Part model, mm, in its own coordinate system. Face numbers are marked on the shaded views. A direction names the side the tool comes from. Coordinates: 2 decimals unless noted, no trailing zeros. Write each loop counter-clockwise with the first axis right and the second up, starting at its lowest first coordinate (ties: lowest second). Pieces come first, ordered by that corner, then holes. Notation, with made-up numbers: (5.5, 9.25) -> (9.5, 9.25) arc R21 ccw to (9.5, 32.25) -> close; hole circle Ø7 at (55, -38.75). An arc over 180 degrees is marked (long way). Write item = value, one per line.
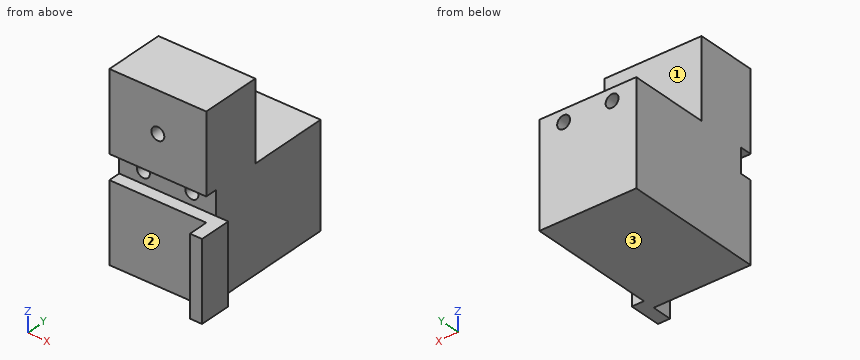
Autodesk Inventor part; units mm, degrees
ref_plane "YZ Plane" through (0, 0, 0) normal (1, 0, 0) x (0, 1, 0)
ref_plane "XZ Plane" through (0, 0, 0) normal (0, 1, 0) x (-1, 0, 0)
ref_plane "XY Plane" through (0, 0, 0) normal (0, 0, 1) x (1, 0, 0)
sketch "Sketch2" plane through (0, 0, 0) normal (0, 1, 0) x (-1, 0, 0)
  line L0 (12, 22.5) -> (-12, 22.5)
  line L1 (-12, 22.5) -> (-12, -22.5)
  line L2 (-12, -22.5) -> (12, -22.5)
  line L3 (12, -22.5) -> (12, 22.5)
  line L4 (12, 22.5) -> (12, 12.5)
  line L5 (12, 12.5) -> (0, 12.5)
  circle A0 centre (0, 12.5) radius 1.6
  line L6 (0, 12.5) -> (0, 0)
  line L7 (0, 0) -> (-6, 0)
  line L8 (-6, 0) -> (6, 0)
  circle A1 centre (-6, 0) radius 1.6
  circle A2 centre (6, 0) radius 1.6
  line L9 (-12, 22.5) -> (12, 22.5)
  line L10 (12, 22.5) -> (12, 0)
  line L11 (12, 0) -> (-12, 0)
  line L12 (-12, 0) -> (-12, 22.5)
  line L13 (-12, 22.5) -> (12, 22.5)
  line L14 (12, 22.5) -> (12, 2.2056)
  line L15 (12, 2.2056) -> (-12, 2.2056)
  line L16 (-12, 2.2056) -> (-12, 22.5)
  dimension "d0" = 24
  dimension "d1" = 45
  dimension "d2" = 10
  dimension "d3" = 3.2
  dimension "d6" = 6
  dimension "d7" = 3.2
  dimension "d8" = 3.2
extrude "Extrusion1" add sketch "Sketch2" along normal blind 35 contours L3 L5 A0 L6 L15 L1 L0 | L3 L15 L6 A0 L5 | L15 L6 L7 A1 L11 L1 | L3 L11 A2 L8 L6 L15 | L11 A1 L7 L8 A2 L3 L2 L1 | L11 L7 A1 | A1 L7 L11 | L11 L8 A2 | A2 L8 L11
sketch "Sketch3" plane through (0, 0, 0) normal (0, -1, 0) x (1, 0, 0)
  line L0 (12, 22.5) -> (12, -22.5)
  line L1 (-12, -22.5) -> (-12, 22.5)
  line L2 (12, 3) -> (-12, 3)
  line L3 (-12, 3) -> (-12, -3)
  line L4 (-12, -3) -> (12, -3)
  line L5 (12, -3) -> (12, 3)
  point P0 (0, 0)
  dimension "d9" = 6
extrude "Extrusion2" cut sketch "Sketch3" against normal blind 3
hole "Hole1" at (-6, 0, 0) at (6, 0, 0) direction (0, 1, 0) diameter 3.2 depth 44.75 countersink diameter 4 countersink angle 90
sketch "Sketch4" plane through (0, 35, 0) normal (0, 1, 0) x (1, 0, 0)
  line L0 (12, -3) -> (12, 3)
  line L1 (-12, -22.5) -> (12, -22.5)
  line L2 (12, -22.5) -> (12, -3)
  line L3 (12, -3) -> (-12, -3)
  line L4 (-12, -3) -> (-12, -22.5)
  point P0 (0, 0)
extrude "Extrusion3" cut sketch "Sketch4" against normal blind 20
sketch "Sketch5" plane through (12, 0, -22.5) normal (1, 0, 0) x (0, 0, -1)
  line L0 (-45, 0) -> (-25.5, 0)
  line L1 (-45, 0) -> (-45, 15)
  line L2 (-25.5, 0) -> (-45, 0)
  line L3 (-45, 0) -> (-45, 3)
  line L4 (-45, 3) -> (-25.5, 3)
  line L5 (-25.5, 3) -> (-25.5, 0)
  point P0 (-22.5, 0)
  dimension "d21" = 3
extrude "Extrusion4" add sketch "Sketch5" along normal blind 3
sketch "Sketch6" plane through (0, 0, 0) normal (0, -1, 0) x (1, 0, 0)
  line L0 (-12, 3) -> (15, 3)
  line L1 (12, 22.5) -> (12, 3)
  line L2 (15, 3) -> (12, 3)
  line L3 (12, 3) -> (12, 22.5)
  line L4 (12, 22.5) -> (15, 22.5)
  line L5 (15, 22.5) -> (15, 3)
  point P0 (0, 0)
extrude "Extrusion5" add sketch "Sketch6" along normal blind 5
sketch "Sketch7" plane through (-12, 0, 3) normal (0, 0, -1) x (-1, 0, 0)
  line L0 (-24, 0) -> (-24, -5)
  line L1 (-27, 3) -> (-27, -5)
  line L2 (-24, -5) -> (-27, -5)
  line L3 (-27, -5) -> (-27, 3)
  line L4 (-27, 3) -> (-24, 3)
  line L5 (-24, 3) -> (-24, -5)
  point P0 (-12, 0)
extrude "Extrusion6" add sketch "Sketch7" along normal blind 25.5
sketch "Sketch8" plane through (-12, 15, 22.5) normal (0, 0, 1) x (1, 0, 0)
  line L0 (27, -12) -> (27, -20)
  line L1 (24, -12) -> (24, -15)
  line L2 (27, -20) -> (24, -20)
  line L3 (24, -20) -> (24, -12)
  line L4 (24, -12) -> (27, -12)
  line L5 (27, -12) -> (27, -20)
  point P0 (12, -15)
extrude "Extrusion7" cut sketch "Sketch8" against normal blind 25.5
properties part number "spoutstandsupport"
Q1. Saw through at A-A on z = 12.5. Give the cut face in (x, y).
Model answer:
outline = (-12, 0) -> (-1.6, 0) -> (-1.6, 15) -> (-12, 15) -> close; (1.6, 0) -> (12, 0) -> (12, 15) -> (1.6, 15) -> close
Q2. Saw through at C-C on z = 0. Give the cut face in (x, y), and give its area (3 significant figures).
Model answer:
outline = (-12, 3) -> (-7.6, 3) -> (-7.6, 35) -> (-12, 35) -> close; (-4.4, 3) -> (4.4, 3) -> (4.4, 35) -> (-4.4, 35) -> close; (7.6, 3) -> (12, 3) -> (12, 35) -> (7.6, 35) -> close
area = 563 mm²
Q3. Probe line 1 (X direction, y = 14, z = 0); line 2 (Z direction, x = 6, y = 22); line 3 (X direction, y = 11.5, z = -6). List the from-to ranges inside material, lowest first. Write a range as from..to.
Model answer:
line_1 = -12..-7.6, -4.4..4.4, 7.6..12
line_2 = -22.5..-1.6, 1.6..3
line_3 = -12..12
Q4. Pin check, flat tips, straight feed: pin 1 (10 mm diameter, centred on x = 3, z = 10, fed in from +Y); pin 2 (3 mm diameter, centred on y = 14, z = 12.5, fed in from +X); pin 3 (5 mm diameter, centred on x = 6, z = 0, fed in from -Y). Stop position of each tip, or through.
Model answer:
pin_1 = 15
pin_2 = 12
pin_3 = 3
Q5. Saw through at B-B on x = 6. Give the cut face in (y, z), and give its area (3 significant figures).
Model answer:
outline = (0, -22.5) -> (35, -22.5) -> (35, -1.6) -> (3, -1.6) -> (3, -3) -> (0, -3) -> close; (0, 3) -> (3, 3) -> (3, 1.6) -> (35, 1.6) -> (35, 3) -> (15, 3) -> (15, 22.5) -> (0, 22.5) -> close
area = 1,060 mm²
Q6. Which spindle directions (+Z, -Z, +X, -X, +Y, -Y) get a long thin tool onto all of the face, cutting with end or side? Do the marked faces 1, 2 and 3. Say none if no direction does.
Model answer:
face_1 = +Z, +X, -X, +Y
face_2 = +Z, -Z, -X, -Y
face_3 = -Z, +X, -X, +Y, -Y
Q7. Saw through at D-D on y = 10.5. Give the cut face in (x, z).
Model answer:
outline = (-12, -22.5) -> (12, -22.5) -> (12, 22.5) -> (-12, 22.5) -> close; hole circle Ø3.2 at (-6, 0); hole circle Ø3.2 at (0, 12.5); hole circle Ø3.2 at (6, 0)
